Check sheet for the modelled part. Datum: model origin and axes. Units: mm. Give positions to 0.01 mm unless a question says otherwise; leave off trailing zeros. Order: outer loops, then holes, each group sorted by start corner. A loop starts at its lowest first (then second) coordinate and runs counter-clockwise, first axis right, second up. Notation, with made-up numbers: (50.5, 73) -> (84.5, 73) arc R20 ccw to (84.5, 91) -> close; hole circle Ø2 at (70, 30). An arc over 180 degrees is marked (long way). One line per question, with ' | ' between items.
```python
from build123d import *

# Parameters (mm, degrees)
EXTRUDE_THIN1_DEPTH = 82.55
SKETCH2_R           = 2.413
CUT_EXTRUDE1_DEPTH  = 3.286
LPATTERN1_COUNT     = 13
LPATTERN1_PITCH     = 12.7
FILLET1_R           = 6.35
SKETCH3_R           = 2.413
CUT_EXTRUDE2_DEPTH  = 3.286
LPATTERN2_COUNT     = 3
LPATTERN2_PITCH     = 76.2
CUT_EXTRUDE3_DEPTH  = 3.286


with BuildPart() as part:
    # Sketch1 → Extrude-Thin1 (new body, symmetric)
    with BuildSketch(Plane(origin=(0, 0, 0), x_dir=(0, 0, -1), z_dir=(1, 0, 0))):
        with BuildLine():
            Line((0, 0), (13.208, 0))
            ThreePointArc((13.208, 0), (16.440892204, 1.339107796), (17.78, 4.572))
            Line((17.78, 4.572), (17.78, 17.78))
            Line((17.78, 17.78), (15.494, 17.78))
            Line((15.494, 17.78), (15.494, 4.572))
            ThreePointArc((15.494, 4.572), (14.824446102, 2.955553898), (13.208, 2.286))
            Line((13.208, 2.286), (0, 2.286))
            Line((0, 2.286), (0, 0))
        make_face()
    extrude(amount=EXTRUDE_THIN1_DEPTH, both=True)

    # Sketch2 → Cut-Extrude1 (cut, through all)
    with BuildSketch(Plane(origin=(0, 2.286, 0), x_dir=(1, 0, 0), z_dir=(0, 1, 0))):
        with Locations((-76.2, 6.35)):
            Circle(SKETCH2_R)
    cut_extrude1 = extrude(amount=-CUT_EXTRUDE1_DEPTH, mode=Mode.SUBTRACT)

    # LPattern1: Cut-Extrude1 ×13
    with Locations(*[(i * LPATTERN1_PITCH, 0, 0) for i in range(1, LPATTERN1_COUNT)]):
        add(cut_extrude1, mode=Mode.SUBTRACT)

    # Fillet1
    fillet1_edges = [part.edges().sort_by_distance(p)[0] for p in [
        (82.55, 1.143, 0),
        (82.55, 17.78, -16.637),
        (-82.55, 1.143, 0),
        (-82.55, 17.78, -16.637),
    ]]
    fillet(fillet1_edges, radius=FILLET1_R)

    # Sketch3 → Cut-Extrude2 (cut, through all)
    with BuildSketch(Plane.XY.offset(-15.494)):
        with Locations((-76.2, 11.43)):
            Circle(SKETCH3_R)
    cut_extrude2 = extrude(amount=-CUT_EXTRUDE2_DEPTH, mode=Mode.SUBTRACT)

    # LPattern2: Cut-Extrude2 ×3
    with Locations(*[(i * LPATTERN2_PITCH, 0, 0) for i in range(1, LPATTERN2_COUNT)]):
        add(cut_extrude2, mode=Mode.SUBTRACT)

    # Sketch4 → Cut-Extrude3 (cut, through all)
    with BuildSketch(Plane.XY.offset(-15.494)):
        with BuildLine():
            Line((-63.5, 13.843), (-12.7, 13.843))
            ThreePointArc((-12.7, 13.843), (-10.287, 11.43), (-12.7, 9.017))
            Line((-12.7, 9.017), (-63.5, 9.017))
            ThreePointArc((-63.5, 9.017), (-65.913, 11.43), (-63.5, 13.843))
        make_face()
        with BuildLine():
            Line((63.5, 13.843), (12.7, 13.843))
            ThreePointArc((12.7, 13.843), (10.287, 11.43), (12.7, 9.017))
            Line((12.7, 9.017), (63.5, 9.017))
            ThreePointArc((63.5, 9.017), (65.913, 11.43), (63.5, 13.843))
        make_face()
    extrude(amount=-CUT_EXTRUDE3_DEPTH, mode=Mode.SUBTRACT)


solid = part.part
```
Q1. Section check C-C (x = 6). Enter the section's corners in (y, z), and give its area (3 significant figures).
Result sheet:
outline: (0, -13.21) arc R4.57 ccw to (4.57, -17.78) -> (17.78, -17.78) -> (17.78, -15.49) -> (4.57, -15.49) arc R2.29 cw to (2.29, -13.21) -> (2.29, 0) -> (0, 0) -> close | area: 72.7 mm2
Q2. Section check D-D (z = -11). Enter the section's corners in (x, y), and give its area (3 significant figures).
Result sheet:
outline: (-82.55, 0) -> (82.55, 0) -> (82.55, 2.29) -> (-82.55, 2.29) -> close | area: 377 mm2
Q3. Mould release check, pull along Y, two halves, no side actions. Record for faces 1 (the face through (80.64, 1.13, -1.81)), 2 (the face through (1.113, 9.289, -16.621)), 3 (the face through (1, 2.286, -10)): pulls with the +Y half, pulls with the -Y half, needs draft (parallel to the pull), parting line crosses it, or undercut.
Result sheet:
face 1: needs draft | face 2: undercut | face 3: pulls with the +Y half
Q4. Depth check by flat-ended pin: pin 1 Ø7.5 at (x, y) = (-76.2, 11.43) entering from +Z; pin 2 Ø7.5 at (x, z) = (63.5, -6.35) entering from +Y; pin 3 Ø1.1 at (x, z) = (-36.5, -17) entering from -Y. Enter the tip coordinate at first touch or a pass-through.
Result sheet:
pin 1: stops at z = -15.49 | pin 2: stops at y = 2.29 | pin 3: stops at y = 1.35
Q5. Section check A-A (x = 38.1). Enter the section's corners in (y, z).
Result sheet:
outline: (0, -13.21) arc R4.57 ccw to (4.57, -17.78) -> (9.02, -17.78) -> (9.02, -15.49) -> (4.57, -15.49) arc R2.29 cw to (2.29, -13.21) -> (2.29, -8.76) -> (0, -8.76) -> close; (0, -3.94) -> (2.29, -3.94) -> (2.29, 0) -> (0, 0) -> close; (13.84, -17.78) -> (17.78, -17.78) -> (17.78, -15.49) -> (13.84, -15.49) -> close
Q6. Thickness scan on line 1 (Y direction, x = -15, z = -2.5); line 2 (Z direction, x = 37.5, y = 16); line 3 (Z direction, x = 63.5, y = 1.7). Record the ranges inside material, lowest first.
Result sheet:
line 1: y = 0 to 2.29 | line 2: z = -17.78 to -15.49 | line 3: z = -16.77 to -8.76, -3.94 to 0
Q7. Section check B-B (x = -44.5). Enter the section's corners in (y, z).
Result sheet:
outline: (0, -13.21) arc R4.57 ccw to (4.57, -17.78) -> (9.02, -17.78) -> (9.02, -15.49) -> (4.57, -15.49) arc R2.29 cw to (2.29, -13.21) -> (2.29, 0) -> (0, 0) -> close; (13.84, -17.78) -> (17.78, -17.78) -> (17.78, -15.49) -> (13.84, -15.49) -> close
